Autodesk Inventor part; units mm, degrees
ref_plane "YZ Plane" through (0, 0, 0) normal (1, 0, 0) x (0, 1, 0)
ref_plane "XZ Plane" through (0, 0, 0) normal (0, 1, 0) x (-1, 0, 0)
ref_plane "XY Plane" through (0, 0, 0) normal (0, 0, 1) x (1, 0, 0)
sketch "Sketch1" plane through (0, 0, 0) normal (0, 0, 1) x (1, 0, 0)
  line L0 (-5.7947, 5.8302) -> (7.2053, 5.8302)
  line L1 (7.2053, 5.8302) -> (7.2053, -7.1698)
  line L2 (7.2053, -7.1698) -> (-5.7947, -7.1698)
  line L3 (-5.7947, -7.1698) -> (-5.7947, 5.8302)
  arc A0 (-5.7947, -7.1698) -> (-1.7947, 5.8302) centre (-34.6583, 8.8267) ccw
  arc A1 (3.2053, 5.8302) -> (7.2053, -7.1698) centre (36.069, 8.8267) ccw
  point P0 (0, 0)
  dimension "d0" = 13
  dimension "d1" = 13
  dimension "d2" = 4
  dimension "d3" = 4
  dimension "d4" = 33
  dimension "d5" = 33
extrude "Extrusion1" add sketch "Sketch1" along normal blind 8.976 contours L0 A1 L2 A0
sketch "Sketch2" plane through (-5.7947, -7.1698, 0) normal (0, -1, 0) x (1, 0, 0)
  line L0 (9.1, 5.188) -> (3.9, 5.188)
  line L1 (3.9, 5.188) -> (3.9, 3.788)
  line L2 (3.9, 3.788) -> (9.1, 3.788)
  line L3 (9.1, 3.788) -> (9.1, 5.188)
  line L4 (0, 8.976) -> (13, 8.976)
  line L5 (13, 0) -> (13, 8.976)
  point P0 (5.7947, 0)
  dimension "d8" = 1.4
  dimension "d9" = 5.2
  dimension "d10" = 3.788
  dimension "d11" = 3.9
extrude "Extrusion2" cut sketch "Sketch2" against normal blind 2
sketch "Sketch3" plane through (-5.7947, -5.1698, 0) normal (0, -1, 0) x (1, 0, 0)
  line L0 (9.1, 3.788) -> (3.9, 3.788)
  line L1 (4.3, 5.188) -> (8.7, 5.188)
  line L2 (8.7, 5.188) -> (8.7, 3.788)
  line L3 (8.7, 3.788) -> (4.3, 3.788)
  line L4 (4.3, 3.788) -> (4.3, 5.188)
  line L5 (3.9, 5.188) -> (9.1, 5.188)
  line L6 (3.9, 3.788) -> (3.9, 5.188)
  line L7 (9.1, 5.188) -> (9.1, 3.788)
  point P0 (5.7947, 0)
  dimension "d14" = 0
  dimension "d15" = 0.4
  dimension "d16" = 0.4
extrude "Extrusion3" cut sketch "Sketch3" against normal blind 10 contours L0 L4 L1 L2
fillet "Fillet1" radius 1 8 edges at (3.2053, 5.8302, 4.488) (-3.1176, -0.8781, 8.976) (0.7053, 5.8302, 8.976) (-1.7947, 5.8302, 4.488) (0.7053, 5.8302, 0) (4.5283, -0.8781, 0) (-3.1176, -0.8781, 0) (4.5283, -0.8781, 8.976)
properties part number "SingleSliderCap"
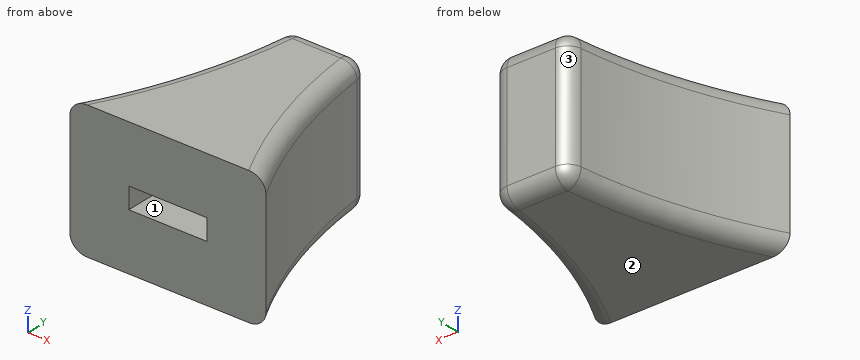
Source: CAD feature listing. Evaluate the final solid. Frame: model axes, mm. Face numbers are marked on the shaded views. Give positions to 0.01 mm unless a question says otherwise; leave off trailing zeros. Order: outer loops, then holes, each group sorted by start corner. A loop starts at its lowest first (then second) coordinate and runs counter-clockwise, first axis right, second up.
(1) Pull-direction query (X, two-part tool) for the marked faces 1, 2 and 3; classes: +X half, -X half, draft (parallel to the pull), parting line (faces both ways), or undercut.
(2) Section query B-B (z = 5). Return the cut outline in (x, y).
(3) Contact query for flat-ended pins moving along their axis: P1, Ø1.5, axis at y = 2, z = 5.5, coming from the -X side; P2, Ø1, axis at y = 4.5, z = 8, coming from the +X side; P3, Ø1.5, axis at y = -5.5, z = 4.5, coming from the +X side. Output: stop coordinate, or through.
(4) Section query A-A (z = 3.5). Return the cut outline in (x, y), plus the area to 3 significant figures.
(5) Material intervals for line 1 along Z through (x, y) = (-0.75, -3); line 2 along X through (y, z) = (-1.5, 4.5); line 3 along Y through (x, z) = (5.75, 6.25), sorted ascending.
Outcome:
1. face 1: undercut
1. face 2: draft
1. face 3: -X half
2. outline: (-5.79, -7.17) - (-1.89, -7.17) - (-1.89, -5.17) - (-1.49, -5.17) - (-1.49, 4.83) - (2.91, 4.83) - (2.91, -5.17) - (3.31, -5.17) - (3.31, -7.17) - (7.21, -7.17) arc R33 cw to (3.3, 4.95) arc R1 ccw to (2.3, 5.83) - (-0.89, 5.83) arc R1 ccw to (-1.89, 4.95) arc R33 cw to start
3. P1: stops at x = -2.54
3. P2: stops at x = 3.42
3. P3: stops at x = 6.71
4. outline: (-5.79, -7.17) - (7.21, -7.17) arc R33 cw to (3.3, 4.95) arc R1 ccw to (2.3, 5.83) - (-0.89, 5.83) arc R1 ccw to (-1.89, 4.95) arc R33 cw to start
4. area: 104 mm2
5. line 1: z = 0 to 3.79, 5.19 to 8.98
5. line 2: x = -3.32 to -1.49, 2.91 to 4.73
5. line 3: y = -7.17 to -4.2
